CAD build for the part. Positions are in the model's coordinates, mm. A direction names the side the tool comes from. Coordinates: 2 decimals unless noted, no trailing zeros. Order: outer loops, then holes, each group sorted by start corner. A loop starts at its lowest first (then second) coordinate and runs counter-clockwise, first axis right, second up.
from build123d import *

# Parameters (mm, degrees)
F0_R     = 74.9064703826
F1_DEPTH = 1.778
F2_W     = 154.2756035924
F2_H     = 153.531037271
F3_DEPTH = 5.13641
F4_T     = 2.5


with BuildPart() as f1:
    # F0 (on Top) → F1 (new body)
    with BuildSketch(Plane.XY):
        Circle(F0_R)
    extrude(amount=F1_DEPTH)

    # F2 (on Top) → F3 (join)
    with BuildSketch(Plane.XY):
        with Locations((0.2817176282, -0.1181550324)):
            Rectangle(F2_W, F2_H)
    extrude(amount=F3_DEPTH)

    # F4
    f4_openings = [f1.faces().sort_by_distance(p)[0] for p in [
        (0.281718, -76.883674, 2.568205),
    ]]
    offset(amount=F4_T, openings=f4_openings, kind=Kind.INTERSECTION)


solid = f1.part
1) Drill centre lines: probe 1 along X at (y, z) = (30.5, 2.25); probe 2 along Z at (x, y) = (15, 46.5); probe 3 along Y at (x, z) = (-17, 2.75). Where is each one in solid material? Low to high.
2) Two-plate mould, pull along Z, no slides. Class faces 3 (the flat face through (-79.356, 0, 2)), 4 (the flat face through (-1, 2, 7.636)), 5 (the flat face through (-1, 1, 5.136)): released by +Z, released by -Z, zero draft, split by the parting line, or undercut.
3) Pin check, flat tip, straight feed: P1, Ø1.5, axis at x = 33.5, z = 2, coming from the -Y side. Stop position of the tip, or through.
4) Slice it at B-B (z = 2.5). List the corners of the cut face in (x, y), plus the area to 3 significant figures.
5) Slice it at A-A (y = -16.5). List the corners of the cut face in (x, z), plus the area to 3 significant figures.
6) Slice it at C-C (x = 22.5). List the corners of the cut face in (y, z), plus the area to 3 significant figures.
7) Which spindle directions (+Z, -Z, +X, -X, +Y, -Y) get a long thin tool onto all of the face, cutting with end or side? Do faces 1 (the flat face through (-1, 76.647, 3)), 2 (the flat face through (-1, -76.884, -1)). Say none if no direction does.
Worked out:
1. probe 1: x = -79.36 to -76.86, 77.42 to 79.92
1. probe 2: z = -2.5 to 0, 5.14 to 7.64
1. probe 3: y = 76.65 to 79.15
2. face 3: zero draft
2. face 4: released by +Z
2. face 5: undercut
3. P1: stops at y = 76.65
4. outline: (-79.36, -76.88) - (-76.86, -76.88) - (-76.86, 76.65) - (77.42, 76.65) - (77.42, -76.88) - (79.92, -76.88) - (79.92, 79.15) - (-79.36, 79.15) - close
4. area: 1,170 mm2
5. outline: (-79.36, -2.5) - (79.92, -2.5) - (79.92, 7.64) - (-79.36, 7.64) - close; hole (-76.86, 0) - (77.42, 0) - (77.42, 5.14) - (-76.86, 5.14) - close
5. area: 822 mm2
6. outline: (-76.88, -2.5) - (79.15, -2.5) - (79.15, 7.64) - (-76.88, 7.64) - (-76.88, 5.14) - (76.65, 5.14) - (76.65, 0) - (-76.88, 0) - close
6. area: 793 mm2
7. face 1: -Y
7. face 2: +Z, -Z, +X, -X, -Y
